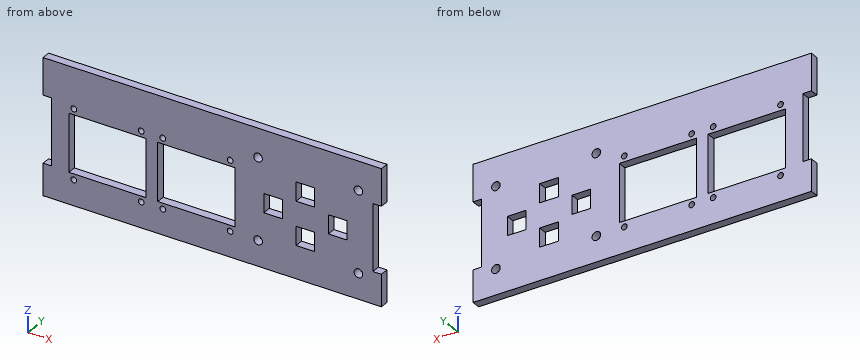
from build123d import *

# Parameters (mm, degrees)
SKETCH1_R           = 1.5
SKETCH1_R_2         = 1
SKETCH1_W           = 27
SKETCH1_H           = 20
SKETCH1_W_2         = 6.5
SKETCH1_H_2         = 6.5
BOSS_EXTRUDE1_DEPTH = 3


with BuildPart() as part:
    # Sketch1 → Boss-Extrude1 (new body)
    with BuildSketch(Plane(origin=(0, 0, 0), x_dir=(1, 0, 0), z_dir=(0, 1, 0))):
        Polygon((-55.548227769, -6.151360111), (-52.548227769, -6.151360111), (-52.548227769, 16.848639889), (-55.548227769, 16.848639889), (-55.548227769, 27.848639889), (62.451772231, 27.848639889), (62.451772231, 16.848639889), (59.451772231, 16.848639889), (59.451772231, -6.151360111), (62.451772231, -6.151360111), (62.451772231, -18.881360111), (-55.548227769, -18.881360111), align=None)
        with Locations(Location((19.451772231, 19.069293812, 0), (0, 0, 270))):
            Circle(SKETCH1_R, mode=Mode.SUBTRACT)
        with Locations(Location((54.451772231, 19.069293812, 0), (0, 0, 270))):
            Circle(SKETCH1_R, mode=Mode.SUBTRACT)
        with Locations(Location((54.451772231, -8.930706188, 0), (0, 0, 270))):
            Circle(SKETCH1_R, mode=Mode.SUBTRACT)
        with Locations(Location((19.451772231, -8.930706188, 0), (0, 0, 270))):
            Circle(SKETCH1_R, mode=Mode.SUBTRACT)
        with Locations(Location((9.701772231, 19.069293812, 0), (0, 0, 270))):
            Circle(SKETCH1_R_2, mode=Mode.SUBTRACT)
        with Locations(Location((9.701772231, -4.930706188, 0), (0, 0, 270))):
            Circle(SKETCH1_R_2, mode=Mode.SUBTRACT)
        with Locations(Location((-13.798227769, -4.930706188, 0), (0, 0, 270))):
            Circle(SKETCH1_R_2, mode=Mode.SUBTRACT)
        with Locations(Location((-13.798227769, 19.069293812, 0), (0, 0, 270))):
            Circle(SKETCH1_R_2, mode=Mode.SUBTRACT)
        with Locations(Location((-44.798227769, 19.069293812, 0), (0, 0, 270))):
            Circle(SKETCH1_R_2, mode=Mode.SUBTRACT)
        with Locations(Location((-21.298227769, 19.069293812, 0), (0, 0, 270))):
            Circle(SKETCH1_R_2, mode=Mode.SUBTRACT)
        with Locations(Location((-44.798227769, -4.930706188, 0), (0, 0, 270))):
            Circle(SKETCH1_R_2, mode=Mode.SUBTRACT)
        with Locations(Location((-21.298227769, -4.930706188, 0), (0, 0, 270))):
            Circle(SKETCH1_R_2, mode=Mode.SUBTRACT)
        with Locations((-2.048227769, 7.069293812)):
            Rectangle(SKETCH1_W, SKETCH1_H, mode=Mode.SUBTRACT)
        with Locations((-33.048227769, 7.069293812)):
            Rectangle(SKETCH1_W, SKETCH1_H, mode=Mode.SUBTRACT)
        with Locations((35.951772231, 13.319293812)):
            Rectangle(SKETCH1_W_2, SKETCH1_H_2, mode=Mode.SUBTRACT)
        with Locations((47.201772231, 5.819293812)):
            Rectangle(SKETCH1_W_2, SKETCH1_H_2, mode=Mode.SUBTRACT)
        with Locations((35.951772231, -1.680706188)):
            Rectangle(SKETCH1_W_2, SKETCH1_H_2, mode=Mode.SUBTRACT)
        with Locations((24.701772231, 5.819293812)):
            Rectangle(SKETCH1_W_2, SKETCH1_H_2, mode=Mode.SUBTRACT)
    extrude(amount=BOSS_EXTRUDE1_DEPTH)


solid = part.part
Design review of the part built by this model. Coordinates are the model's own, in mm. Give positions to 0.01 mm unless a question says otherwise; leave off trailing zeros. Loops run counter-clockwise (first coordinate to the right, second up) from the corner with the lowest first, then second, coordinate; pieces in that order, holes last. Notation, with made-up numbers: M 26,87.25 L 42,87.25 A26 cw 42,122.25 Z; hole C 5.25,42.5 d7. An arc over 180 degrees is marked long. Answer as a JSON object with one key per item and string values.
Item 1: Wall thickness on line 1 along X through (y, z) = (1.6, -2); line 2 along X through (y, z) = (0.5, 9); line 3 along X through (y, z) = (0.9, -11.5): over which ranges is each line inside the solid? List them lowest first.
Output values:
{"line 1": "x = -52.55 to -46.55, -19.55 to -15.55, 11.45 to 59.45", "line 2": "x = -55.55 to 17.95, 20.95 to 52.95, 55.95 to 62.45", "line 3": "x = -52.55 to -46.55, -19.55 to -15.55, 11.45 to 32.7, 39.2 to 59.45"}
Item 2: We need section D-D (x = 38). State the section outline as (y, z) points, and give its area (3 significant figures).
Output values:
{"outline": "M 0,-27.85 L 3,-27.85 L 3,-16.57 L 0,-16.57 Z; M 0,-10.07 L 3,-10.07 L 3,-1.57 L 0,-1.57 Z; M 0,4.93 L 3,4.93 L 3,18.88 L 0,18.88 Z", "area": "101 mm2"}
Item 3: We need section C-C (z = -15.5). State the section outline as (x, y) points.
Output values:
{"outline": "M -52.55,0 L -46.55,0 L -46.55,3 L -52.55,3 Z; M -19.55,0 L -15.55,0 L -15.55,3 L -19.55,3 Z; M 11.45,0 L 32.7,0 L 32.7,3 L 11.45,3 Z; M 39.2,0 L 59.45,0 L 59.45,3 L 39.2,3 Z"}
Item 4: We need section B-B (z = -6). State the section outline as (x, y) points, and give its area (3 significant figures).
Output values:
{"outline": "M -52.55,0 L -46.55,0 L -46.55,3 L -52.55,3 Z; M -19.55,0 L -15.55,0 L -15.55,3 L -19.55,3 Z; M 11.45,0 L 21.45,0 L 21.45,3 L 11.45,3 Z; M 27.95,0 L 43.95,0 L 43.95,3 L 27.95,3 Z; M 50.45,0 L 59.45,0 L 59.45,3 L 50.45,3 Z", "area": "135 mm2"}
Item 5: For P1, Ø0.9, axis at y = 2, z = -4.5, coming from the -X side; P2, Ø2.5, axis at x = 54.45, z = 8.93, coming from the -Y side; P3, Ø1.5, axis at y = 1.5, z = -10, coming from the +X side, all flat-tipped, find the tip position at first contact; note any pin that passes through.
Output values:
{"P1": "stops at x = -52.55", "P2": "passes through", "P3": "stops at x = 59.45"}
Item 6: We need section A-A (x = -33). State the section outline as (y, z) points, and give its area (3 significant figures).
Output values:
{"outline": "M 0,-27.85 L 3,-27.85 L 3,-17.07 L 0,-17.07 Z; M 0,2.93 L 3,2.93 L 3,18.88 L 0,18.88 Z", "area": "80.2 mm2"}
